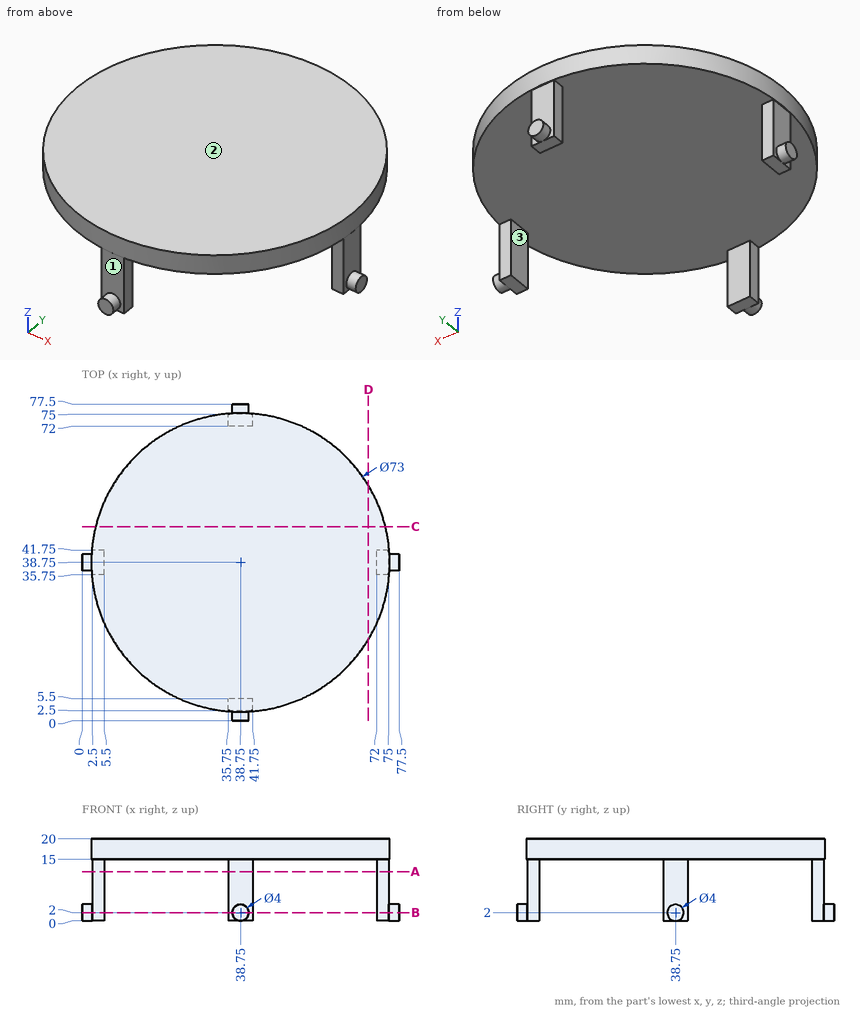
The figure shows three views and two pictorial views of one solid part (mm, origin at its lowest corner). Answer the questions. Give positions to 0.01 mm unless a question says otherwise; leave off trailing zeros. Loops run counter-clockwise (first coordinate to the right, second up) from the corner with the lowest first, then second, coordinate; pieces in that order, holes last. Notation, with made-up numbers: (36.5, -37) -> (70.5, -37) arc R27 cw to (70.5, -12) -> close; hole circle Ø7 at (-3.75, 32.25). An arc over 180 degrees is marked (long way). Put each result on its own line as item: value. Start each with the question number.
Item 1: The mould has two halves that part along Z. Classify the marked faces 1, 2 and 3: released by +Z, released by -Z, zero draft, split by the parting line, or undercut.
Item 2: The part is cut by section C-C (y = 47.5). Give the vertices of the cut face in (x, z), then the cut area to 3 significant figures.
Item 3: The part is cut by section B-B (z = 2). State how many separate pieces and enclosed holes the cut face has, then the cut area to 3 significant figures.
Item 4: The part is cut by section A-A (z = 12). Give the vertices of the cut face in (x, y), then the cut area to 3 significant figures.
Item 5: Find the intervals of material crossed by L1, parallel to X at y = 38, z = 1.75; L2, parallel to Z at x = 60.5, y = 55; L3, parallel to Y at x = 5, z = 6.5, in increasing order. Write a range as [from, to].
Item 6: The part is cut by section D-D (x = 70). Give the vertices of the cut face in (y, z), then the cut area to 3 significant figures.
Item 7: Each of these flat-tipped pins is pushed along its axis until it touches: P1, Ø0.9, axis at x = 3.5, z = 5, coming from the +Y side; P2, Ø3.5, axis at y = 3.5, z = 7, coming from the -X side; P3, Ø5, axis at y = 19, z = 12, coming from the +X side; P4, Ø3.5, axis at x = 4, z = 7, coming from the -Y side. Where does it stop, or does it pass through?
Answers below:
1. face 1: undercut
1. face 2: released by +Z
1. face 3: zero draft
2. outline: (3.31, 15) -> (74.19, 15) -> (74.19, 20) -> (3.31, 20) -> close
2. area: 354 mm2
3. separate pieces: 4
3. enclosed holes: 0
3. area: 112 mm2
4. outline: (2.5, 35.75) -> (5.5, 35.75) -> (5.5, 41.75) -> (2.5, 41.75) -> close; (35.75, 2.5) -> (41.75, 2.5) -> (41.75, 5.5) -> (35.75, 5.5) -> close; (35.75, 72) -> (41.75, 72) -> (41.75, 75) -> (35.75, 75) -> close; (72, 35.75) -> (75, 35.75) -> (75, 41.75) -> (72, 41.75) -> close
4. area: 72.0 mm2
5. L1: [0, 5.5], [72, 77.5]
5. L2: [15, 20]
5. L3: [35.75, 41.75]
6. outline: (19.89, 15) -> (57.61, 15) -> (57.61, 20) -> (19.89, 20) -> close
6. area: 189 mm2
7. P1: y = 41.75
7. P2: x = 35.75
7. P3: through
7. P4: y = 35.75
